Can you work these out from the drawing? Everything is in mm from the part's minimum corner. A direction names the side the tool comes from. Round coordinates to 2 decimals unless told otherwise and drop trailing zeros. Order: outer loops, then holes, each group sorted by start corner. A loop starts at its lowest first (then second) coordinate and runs counter-clockwise, first axis right, second up. Notation, with made-up numbers: (32, 16) -> (63, 16) arc R13 ccw to (63, 36) -> close; hole circle Ø8 at (89, 88). An arc over 180 degrees is marked (long way). Use a Markdown table: item, result. Add a question column.
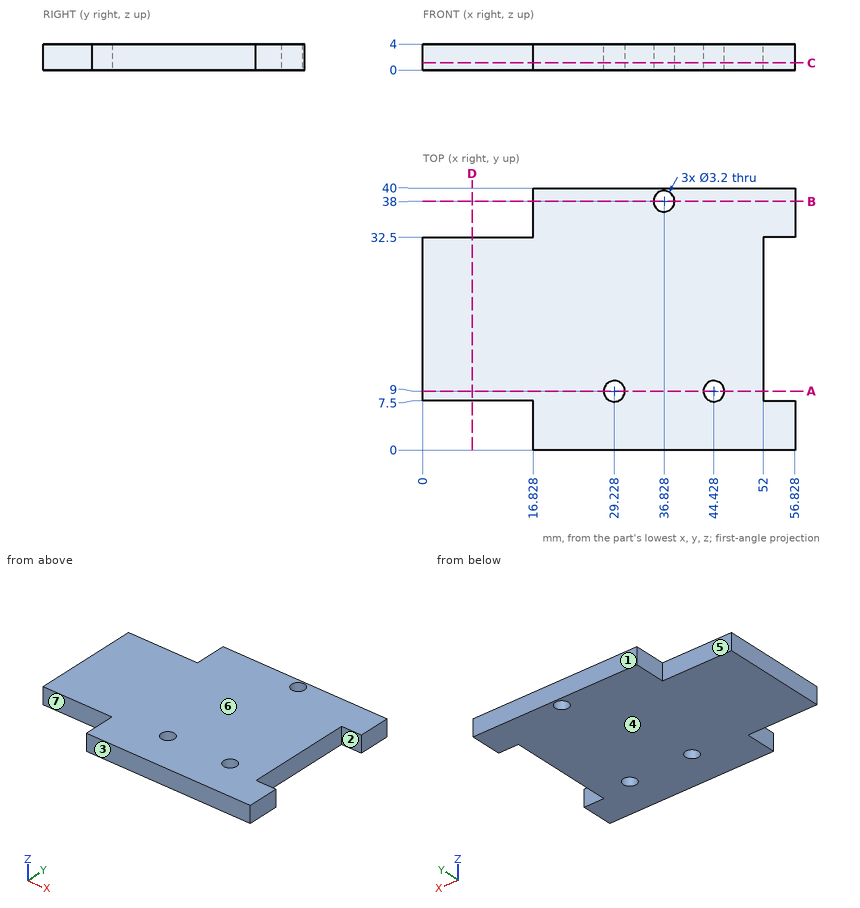
(1) On a 3-axis mill with a long thin cutter (end or side, diameter ignored), from which of +Z, -Z, +X, -X, +Y, -Y can I reach the whole of each face in a straight line? I mean the marked faces 5, 6 and 7. Say none if no direction works.
(2) I'm going to push flat-ended pins straight in: P1, Ø2, axis at y = 4.5, z = 2, coming from the -X side; P2, Ø1.2, axis at x = 5.5, z = 2, coming from the +Y side; P3, Ø2.5, axis at x = 29.23, y = 9, coming from the -Z side. Where does each tip first touch, or does it pass through?
(3) I want a section at A-A on y = 9. List the corners of the cut face in (x, z) for me.
(4) Please list where these lines run through material, in increasing order: probe 1 along X at (y, z) = (9, 3); probe 2 along X at (y, z) = (33, 2.3); probe 3 along X at (y, z) = (29.5, 3.3). Write a range as from..to.
(5) I want a section at D-D on x = 7.5. List the corners of the cut face in (y, z) for me, and give its area (3 significant figures).
(6) I want a section at B-B on y = 38. List the corners of the cut face in (x, z) for me.
(7) If we mould it in two halves opening along Y, with no side actions, what happens to the marked faces 1, 2, 3 and 4? For each: pulls with the +Y half, pulls with the -Y half, needs draft (parallel to the pull), parting line crosses it, or undercut.
(8) I want a section at C-C on z = 1.1. List the corners of the cut face in (x, y) for me.
Output:
| question | item | result |
|---|---|---|
| 1 | face 5 | +Z, -Z, -X, +Y |
| 1 | face 6 | +Z, +X, -X, +Y, -Y |
| 1 | face 7 | +Z, -Z, -X, -Y |
| 2 | P1 | x = 16.83 |
| 2 | P2 | y = 32.5 |
| 2 | P3 | through |
| 3 | outline | (0, 0) -> (27.63, 0) -> (27.63, 4) -> (0, 4) -> close; (30.83, 0) -> (42.83, 0) -> (42.83, 4) -> (30.83, 4) -> close; (46.03, 0) -> (52, 0) -> (52, 4) -> (46.03, 4) -> close |
| 4 | probe 1 | 0..27.63, 30.83..42.83, 46.03..52 |
| 4 | probe 2 | 16.83..56.83 |
| 4 | probe 3 | 0..52 |
| 5 | outline | (7.5, 0) -> (32.5, 0) -> (32.5, 4) -> (7.5, 4) -> close |
| 5 | area | 100 mm² |
| 6 | outline | (16.83, 0) -> (35.23, 0) -> (35.23, 4) -> (16.83, 4) -> close; (38.43, 0) -> (56.83, 0) -> (56.83, 4) -> (38.43, 4) -> close |
| 7 | face 1 | pulls with the +Y half |
| 7 | face 2 | undercut |
| 7 | face 3 | pulls with the -Y half |
| 7 | face 4 | needs draft |
| 8 | outline | (0, 7.5) -> (16.83, 7.5) -> (16.83, 0) -> (56.83, 0) -> (56.83, 7.5) -> (52, 7.5) -> (52, 32.5) -> (56.83, 32.5) -> (56.83, 40) -> (16.83, 40) -> (16.83, 32.5) -> (0, 32.5) -> close; hole circle Ø3.2 at (29.23, 9); hole circle Ø3.2 at (36.83, 38); hole circle Ø3.2 at (44.43, 9) |
